```python
from build123d import *

# Parameters (mm, degrees)
F3_DEPTH = 50
F2_R     = 14.5
F4_DEPTH = 75
F5_DEPTH = 43.9
F6_W     = 29
F6_H     = 29
F7_DEPTH = 59.8


with BuildPart() as f3:
    # F1 (on Top) → F3 (new body)
    with BuildSketch(Plane.XY):
        with BuildLine():
            ThreePointArc((32.19508, 15.206385), (29.266148, 22.277453), (22.19508, 25.206385))
            Line((22.19508, 25.206385), (-22.19508, 25.206385))
            ThreePointArc((-22.19508, 25.206385), (-29.266148, 22.277453), (-32.19508, 15.206385))
            Line((-32.19508, 15.206385), (-32.19508, -16.179468))
            ThreePointArc((-32.19508, -16.179468), (-29.266148, -23.250536), (-22.19508, -26.179468))
            Line((-22.19508, -26.179468), (22.19508, -26.179468))
            ThreePointArc((22.19508, -26.179468), (29.266148, -23.250536), (32.19508, -16.179468))
            Line((32.19508, -16.179468), (32.19508, 15.206385))
        make_face()
    extrude(amount=F3_DEPTH)

    # F2 (on Top) → F4 (cut)
    with BuildSketch(Plane.XY):
        Circle(F2_R)
    extrude(amount=F4_DEPTH, mode=Mode.SUBTRACT)

    # F0 (on Top) → F5 (cut)
    with BuildSketch(Plane.XY):
        with BuildLine():
            Line((23.5, 20), (-23.5, 20))
            Line((-23.5, 20), (-24.497404, 13.350641))
            ThreePointArc((-24.497404, 13.350641), (-25.493132, 0), (-24.497404, -13.350641))
            Line((-24.497404, -13.350641), (-23.5, -20))
            Line((-23.5, -20), (23.5, -20))
            Line((23.5, -20), (24.497404, -13.350641))
            ThreePointArc((24.497404, -13.350641), (25.493132, 0), (24.497404, 13.350641))
            Line((24.497404, 13.350641), (23.5, 20))
        make_face()
    extrude(amount=F5_DEPTH, mode=Mode.SUBTRACT)

    # F6 (on face) → F7 (cut)
    with BuildSketch(Plane.XY.offset(50)):
        with Locations((0, -14.5)):
            Rectangle(F6_W, F6_H)
    extrude(amount=-F7_DEPTH, mode=Mode.SUBTRACT)


solid = f3.part
```
Verification items for the finished model (mm, model axes). A direction names the side the tool comes from. Coordinates: 2 decimals unless noted, no trailing zeros. Loops run counter-clockwise (first coordinate to the right, second up) from the corner with the lowest first, then second, coordinate; pieces in that order, holes last. Notation, with made-up numbers: (42, -4.75) -> (87, -4.75) arc R24 ccw to (87, 24.25) -> close; hole circle Ø5 at (-3.5, 71). An arc over 180 degrees is marked (long way). Answer in a Markdown table with one row per item.
1) Section check C-C (y = -21). Record the cut outline in (x, z).
The answers:
| item | result |
|---|---|
| outline | (-30.96, 0) -> (-14.5, 0) -> (-14.5, 50) -> (-30.96, 50) -> close; (14.5, 0) -> (30.96, 0) -> (30.96, 50) -> (14.5, 50) -> close |
2) Draft check along Y on faces 4 (the face through (32.195, -1, 25)), 5 (the face through (0, 25.206, 25)), 6 (the face through (-25.493, 0.188, 21.643)). Enter one of: released by +Y, released by -Y, zero draft, split by the parting line, or undercut.
The answers:
| item | result |
|---|---|
| face 4 | zero draft |
| face 5 | released by +Y |
| face 6 | undercut |
3) Section check D-D (x = 0). Record the cut outline in (y, z).
The answers:
| item | result |
|---|---|
| outline | (14.5, 43.9) -> (20, 43.9) -> (20, 0) -> (25.21, 0) -> (25.21, 50) -> (14.5, 50) -> close |
4) Section check A-A (x = 21). Record the cut outline in (y, z).
The answers:
| item | result |
|---|---|
| outline | (-26.18, 0) -> (-20, 0) -> (-20, 43.9) -> (20, 43.9) -> (20, 0) -> (25.21, 0) -> (25.21, 50) -> (-26.18, 50) -> close |
5) Section check B-B (z = 15). Record the cut outline in (x, y), and give its area (3 significant figures).
The answers:
| item | result |
|---|---|
| outline | (-32.2, -16.18) arc R10 ccw to (-22.2, -26.18) -> (-14.5, -26.18) -> (-14.5, -20) -> (-23.5, -20) -> (-24.5, -13.35) arc R90 cw to (-24.5, 13.35) -> (-23.5, 20) -> (23.5, 20) -> (24.5, 13.35) arc R90 cw to (24.5, -13.35) -> (23.5, -20) -> (14.5, -20) -> (14.5, -26.18) -> (22.2, -26.18) arc R10 ccw to (32.2, -16.18) -> (32.2, 15.21) arc R10 ccw to (22.2, 25.21) -> (-22.2, 25.21) arc R10 ccw to (-32.2, 15.21) -> close |
| area | 1,060 mm2 |
6) Depth check by flat-ended pin: P1, Ø2, axis at y = -20, z = 34, coming from the -X side; P2, Ø2, axis at x = -4.5, z = 38, coming from the -Y side. Enter the tip coordinate at first touch or a pass-through.
The answers:
| item | result |
|---|---|
| P1 | stops at x = -31.79 |
| P2 | stops at y = 20 |
7) Scan lines: line 1 along Y through (x, z) = (18, 18); line 2 along Y through (x, z) = (-3, 22); line 3 along X through (y, z) = (-5, 47). Record each from-to range of solid material in increasing order. Write a range as from..to.
The answers:
| item | result |
|---|---|
| line 1 | y = -26.18..-20, 20..25.21 |
| line 2 | y = 20..25.21 |
| line 3 | x = -32.2..-14.5, 14.5..32.2 |
8) Access from +Z, -Z, +X, -X, +Y, -Y to the whole of each face (thin tool, end or side, straight path). Record for faces 1 (the face through (-23.99, 16.72, 21.64)), 2 (the face through (14.5, -21, 31)), 3 (the face through (-29.19, 22.35, 24.65)).
The answers:
| item | result |
|---|---|
| face 1 | -Z |
| face 2 | +Z, -Z, -Y |
| face 3 | +Z, -Z, -X, +Y |
